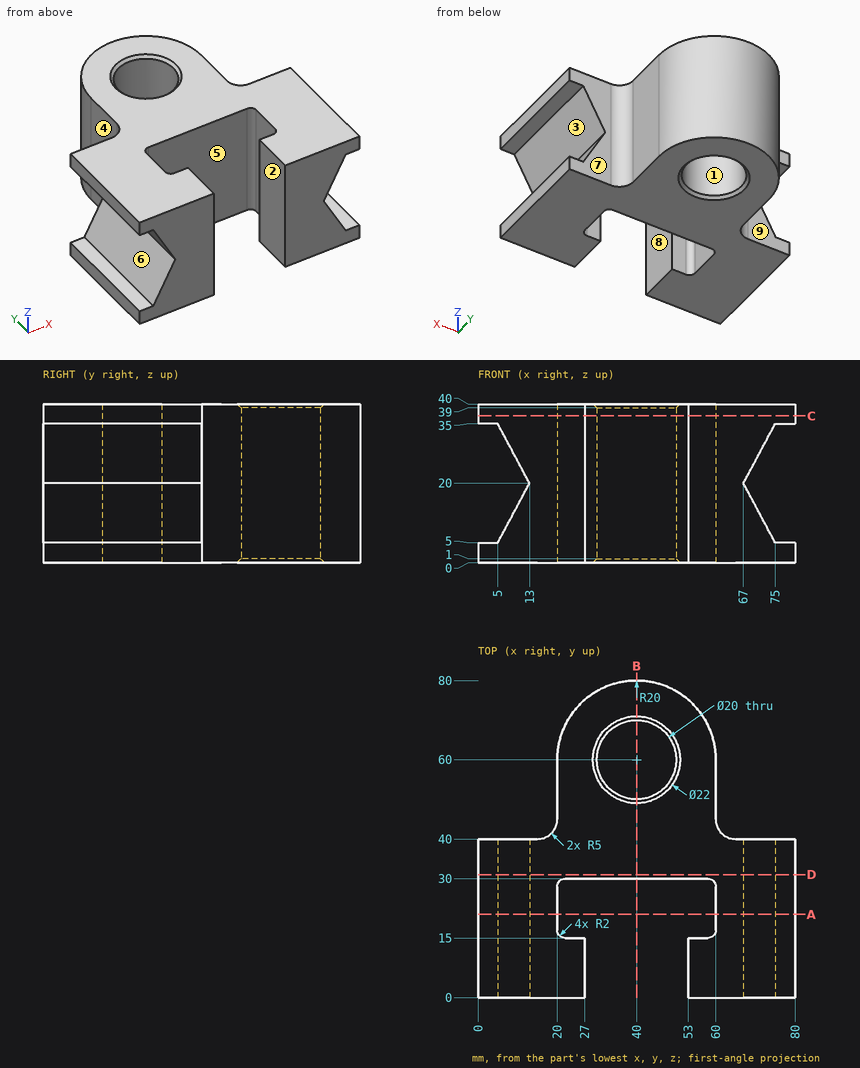
Design review of the part shown in the three views and the two pictorial views. Dimensions are in mm from the part's minimum x, y and z. A direction names the side the tool comes from. Round coordinates to 2 decimals unless told otherwise and drop trailing zeros. Write each loop counter-clockwise with the first axis right and the second up, starting at its lowest first coordinate (ties: lowest second). Pieces come first, ordered by that corner, then holes.
Item 1: The part is to be moulded in two halves that separate along X. For the marked faces 1, 2, 3 and 4, say which applies: +X half, -X half, draft (parallel to the pull), parting line (faces both ways), or undercut.
Item 2: For the marked faces 5, 6, 7, 8 and 9, list the 3-axis set-ups (+Z, -Z, +X, -X, +Y, -Y) from which the entire face can be reached by the end or side of a thin tool; tool diameter is ignored.
Item 3: For probe 1 along Y at (x, z) = (40, 31.5); probe 2 along X at (y, z) = (12.5, 4); probe 3 along Y at (x, z) = (69.5, 10.5), list the stretches that pass through material, from the lowest coordinate up.
Item 4: Clearance check with flat-ended pins moving along their axes: pin 1 Ø12 at (y, z) = (23.5, 18.5) entering from -X; pin 2 Ø1 at (x, z) = (31.5, 27.5) entering from +Y; pin 3 Ø1 at (x, z) = (57, 10.5) entering from +Y; pin 4 Ø4.5 at (x, z) = (4, 28.5) entering from +Y. State where each tip first meets the part, or that it passes through.
Item 5: We need section D-D on y = 31. Write out the cut boundary in (x, z).
Item 6: We need section B-B on x = 40. Write out the cut boundary in (y, z), and give its area (3 significant figures).
Item 7: We need section A-A on y = 21. Write out the cut boundary in (x, z), and give its area (3 significant figures).
Item 8: We need section C-C on z = 37. Write out the cut boundary in (x, y).
Returned:
1. face 1: undercut
1. face 2: undercut
1. face 3: +X half
1. face 4: -X half
2. face 5: +Z, -Z
2. face 6: -X, +Y, -Y
2. face 7: +Z, -Z, +X, +Y
2. face 8: +Z, -Z, -Y
2. face 9: +Z, -Z, -X, +Y
3. probe 1: y = 30 to 50, 70 to 80
3. probe 2: x = 0 to 27, 53 to 80
3. probe 3: y = 0 to 40
4. pin 1: stops at x = 9
4. pin 2: stops at y = 78.33
4. pin 3: stops at y = 71.3
4. pin 4: passes through
5. outline: (0, 0) - (80, 0) - (80, 5) - (75, 5) - (67, 20) - (75, 35) - (80, 35) - (80, 40) - (0, 40) - (0, 35) - (5, 35) - (13, 20) - (5, 5) - (0, 5) - close
6. outline: (30, 0) - (49, 0) - (50, 1) - (50, 39) - (49, 40) - (30, 40) - close; (70, 1) - (71, 0) - (80, 0) - (80, 40) - (71, 40) - (70, 39) - close
6. area: 1,200 mm2
7. outline: (0, 0) - (20, 0) - (20, 40) - (0, 40) - (0, 35) - (5, 35) - (13, 20) - (5, 5) - (0, 5) - close; (60, 0) - (80, 0) - (80, 5) - (75, 5) - (67, 20) - (75, 35) - (80, 35) - (80, 40) - (60, 40) - close
7. area: 1,060 mm2
8. outline: (0, 0) - (27, 0) - (27, 15) - (22, 15) arc R2 cw to (20, 17) - (20, 28) arc R2 cw to (22, 30) - (58, 30) arc R2 cw to (60, 28) - (60, 17) arc R2 cw to (58, 15) - (53, 15) - (53, 0) - (80, 0) - (80, 40) - (65, 40) arc R5 cw to (60, 45) - (60, 60) arc R20 ccw to (20, 60) - (20, 45) arc R5 cw to (15, 40) - (0, 40) - close; hole circle Ø20 at (40, 60)
